Geometry: final body of the model. Coordinates: model frame, mm. Round coordinates to 2 decimals unless told otherwise and drop trailing zeros. Write each loop counter-clockwise with the first axis right and the second up, starting at its lowest first coordinate (ties: lowest second). Pieces come first, ordered by that corner, then holes. Notation, with made-up numbers: M 87.5,58 L 94.5,58 A26 ccw 94.5,95 Z; hole C 41,35.5 d9. An arc over 180 degrees is marked long. Answer as CSV lines item,"result". Start each with the question number.
Q1. Section query C-C on x = 25.4. Output: boundary loops of the cut face in (y, z).
Q2. Ray query, probe 1 along Y at (x, z) = (712, 15.5); probe 2 along Z at (x, y) = (618, 29.5); probe 3 along Y at (x, z) = (25.4, 9.25). Return the intervals inside material, ascending.
Q3. Section query B-B on x = 1664. Output: boundary loops of the cut face in (y, z), and give its area (3 significant figures).
Q4. Section query A-A on z = 21.5. Output: boundary loops of the cut face in (x, y).
Q5. Section query D-D on y = 19. Output: boundary loops of the cut face in (x, z).
Autodesk Inventor part; units mm, degrees
ref_plane "YZ Plane" through (0, 0, 0) normal (1, 0, 0) x (0, 1, 0)
ref_plane "XZ Plane" through (0, 0, 0) normal (0, 1, 0) x (-1, 0, 0)
ref_plane "XY Plane" through (0, 0, 0) normal (0, 0, 1) x (1, 0, 0)
sketch "Sketch3" plane through (0, 0, 0) normal (1, 0, 0) x (0, 1, 0)
  line L0 (36.8031, 29.6629) -> (-6.3261, 29.6629)
  line L1 (-6.3261, 29.6629) -> (-6.3261, 11.9337)
  line L2 (-6.3261, 11.9337) -> (36.8031, 11.9337)
  line L3 (36.8031, 11.9337) -> (36.8031, 29.6629)
  line L4 (40.6385, 33.4983) -> (-10.1615, 33.4983)
  line L5 (-10.1615, 33.4983) -> (-10.1615, 8.0983)
  line L6 (-10.1615, 8.0983) -> (40.6385, 8.0983)
  line L7 (40.6385, 8.0983) -> (40.6385, 33.4983)
  point P0 (0, 0)
  dimension "d2" = 43.1292
  dimension "d3" = 17.7292
  dimension "d4" = 50.8
  dimension "d5" = 25.4
  dimension "d6" = 3.8354
  dimension "d7" = 3.8354
extrude "Extrusion1" add sketch "Sketch3" along normal blind 1828.8
sketch "Sketch4" plane through (0, -10.1615, 33.4983) normal (0, 0, 1) x (1, 0, 0)
  circle A0 centre (25.4, 25.4) radius 14.2875
  line L0 (0, 50.8) -> (1828.8, 50.8)
  line L1 (0, 50.8) -> (0, 0)
  point P0 (0, 10.1615)
  dimension "d10" = 28.575
  dimension "d11" = 25.4
  dimension "d12" = 25.4
hole "Hole1" at (25.4, 15.2385, 33.4983) direction (0, 0, -1) diameter 31.75 end through all
properties part number "box beam"
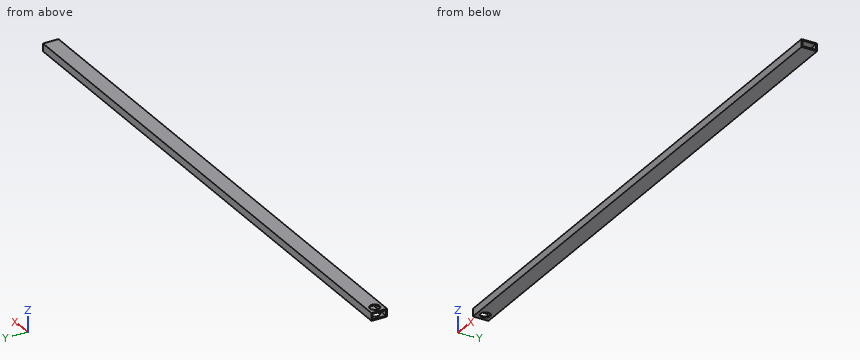
Entries:
1,outline,"M -10.16,8.1 L -0.64,8.1 L -0.64,11.93 L -6.33,11.93 L -6.33,29.66 L -0.64,29.66 L -0.64,33.5 L -10.16,33.5 Z; M 31.11,8.1 L 40.64,8.1 L 40.64,33.5 L 31.11,33.5 L 31.11,29.66 L 36.8,29.66 L 36.8,11.93 L 31.11,11.93 Z"
2,probe 1,"y = -10.16 to -6.33, 36.8 to 40.64"
2,probe 2,"z = 8.1 to 11.93, 29.66 to 33.5"
2,probe 3,"y = -10.16 to -0.64, 31.11 to 40.64"
3,outline,"M -10.16,8.1 L 40.64,8.1 L 40.64,33.5 L -10.16,33.5 Z; hole M -6.33,11.93 L 36.8,11.93 L 36.8,29.66 L -6.33,29.66 Z"
3,area,"526 mm^2"
4,outline,"M 0,-10.16 L 1828.8,-10.16 L 1828.8,-6.33 L 0,-6.33 Z; M 0,36.8 L 1828.8,36.8 L 1828.8,40.64 L 0,40.64 Z"
5,outline,"M 0,8.1 L 9.98,8.1 L 9.98,11.93 L 0,11.93 Z; M 0,29.66 L 9.98,29.66 L 9.98,33.5 L 0,33.5 Z; M 40.82,8.1 L 1828.8,8.1 L 1828.8,11.93 L 40.82,11.93 Z; M 40.82,29.66 L 1828.8,29.66 L 1828.8,33.5 L 40.82,33.5 Z"
